Autodesk Inventor part; units mm, degrees
ref_plane "YZ Plane" through (0, 0, 0) normal (1, 0, 0) x (0, 1, 0)
ref_plane "XZ Plane" through (0, 0, 0) normal (0, 1, 0) x (-1, 0, 0)
ref_plane "XY Plane" through (0, 0, 0) normal (0, 0, 1) x (1, 0, 0)
sketch "Skizze1" plane through (0, 0, 0) normal (0, 0, 1) x (1, 0, 0)
  arc A0 (6, 0) -> (-6, 0) centre (0, 0) ccw
  arc A1 (7.5, 0) -> (-7.5, 0) centre (0, 0) ccw
  arc A2 (-6, -80) -> (6, -80) centre (0, -80) ccw
  line L0 (0, -80) -> (6, -80) construction
  line L1 (0, -80) -> (-6, -80) construction
  arc A3 (-7.5, -80) -> (7.5, -80) centre (0, -80) ccw
  line L2 (0, -80) -> (7.5, -80) construction
  line L3 (0, -80) -> (-7.5, -80) construction
  line L4 (-7.5, -80) -> (-7.5, 0)
  line L5 (-6, 0) -> (-6, -80)
  line L6 (6, -80) -> (6, 0)
  line L7 (7.5, -80) -> (7.5, 0)
  dimension "d0" = 6
  dimension "d1" = 7.5
  dimension "d2" = 6
  dimension "d3" = 180
  dimension "d4" = 7.5
  dimension "d5" = 180
  dimension "d6" = 80
  dimension "d7" = 0
extrude "Extrusion1" add sketch "Skizze1" along normal blind 6
properties part number "Y belt" material "Gummi, Silikon"
Build history of the part. All positions in model axes, mm. A direction names the side the tool comes from. Round coordinates to 2 decimals unless told otherwise and drop trailing zeros. Write each loop counter-clockwise with the first axis right and the second up, starting at its lowest first coordinate (ties: lowest second). Pieces come first, ordered by that corner, then holes. Notation, with made-up numbers: M 55,43.5 L 108,43.5 A27 ccw 108,69.5 Z; hole C -17,22 d5. An arc over 180 degrees is marked long. Answer as a JSON object with one key per item and string values. Group by question number.
(1) Mould opens along Y. For faces 1 (the cylindrical face through (0, 6, 3)), 2 (the flat face through (7.5, -41, 3)), 3 (the cylindrical face through (0.16, -87.5, 2.96)) say: pulls with the +Y half, pulls with the -Y half, needs draft (parallel to the pull), parting line crosses it, or undercut.
(2) Which spindle directions (+Z, -Z, +X, -X, +Y, -Y) get a long thin tool onto all of the face, cutting with end or side? Do faces 4 (the flat face through (6, -41, 3)), 5 (the flat face through (-6.15, -36.26, 0)). Say none if no direction does.
(3) Cut at C-C (z = 1.1). Give the cut face in (x, y).
(4) Flat gauge pin, fed straight in: pin 1 (5 mm diameter, centred on x = -6, y = -33, fed in from -Z). Where does the tip first touch, or does it go through?
(5) Cut at A-A (x = 0). Give the cut face in (y, z), and give its area (3 significant figures).
(6) Drill centre lines: L1, parallel to X at y = -53, z = 4.15; L2, parallel to Y at x = 0, z = 3.15; L3, parallel to Y at x = 1.75, z = 2.05. Where is each one in solid material? Low to high.
(7) Cut at B-B (y = -18.5). Give the cut face in (x, z).
Responses:
{
 "1": {"face 1": "undercut", "face 2": "needs draft", "face 3": "pulls with the -Y half"},
 "2": {"face 4": "+Z, -Z", "face 5": "-Z, +X, -X, +Y, -Y"},
 "3": {"outline": "M -7.5,-80 A7.5 ccw 7.5,-80 L 7.5,0 A7.5 ccw -7.5,0 Z; hole M -6,-80 A6 ccw 6,-80 L 6,0 A6 ccw -6,0 Z"},
 "4": {"pin 1": "stops at z = 0"},
 "5": {"outline": "M -87.5,0 L -86,0 L -86,6 L -87.5,6 Z; M 6,0 L 7.5,0 L 7.5,6 L 6,6 Z", "area": "18.0 mm2"},
 "6": {"L1": "x = -7.5 to -6, 6 to 7.5", "L2": "y = -87.5 to -86, 6 to 7.5", "L3": "y = -87.29 to -85.74, 5.74 to 7.29"},
 "7": {"outline": "M -7.5,0 L -6,0 L -6,6 L -7.5,6 Z; M 6,0 L 7.5,0 L 7.5,6 L 6,6 Z"}
}
